Design review of the part built by this model. Coordinates are the model's own, in mm. A direction names the side the tool comes from. Coordinates: 2 decimals unless noted, no trailing zeros. Loops run counter-clockwise (first coordinate to the right, second up) from the corner with the lowest first, then second, coordinate; pieces in that order, holes last. Notation, with made-up numbers: M -3,14 L 38,14 A19 ccw 38,47 Z; hole C -29,-27 d10. An arc over 180 degrees is marked long. Put each result on its own line as item: value. Start each with the question number.
(1) Take a section at B-B, the plane y = -90. Give the boundary of the cut face in (x, z).
(2) Take a section at A-A, the plane x = 180. Give the boundary of the cut face in (y, z).
(3) For probe 1 along X at (y, z) = (-11.5, 4.5); probe 2 along Y at (x, z) = (-180, 4.75); probe 3 along Y at (x, z) = (0, 2.5), list the stretches that pass through material, from the lowest coordinate up. Write a range as [from, to].
(4) For faces 5 (the flat face through (-3, 2, 8)), 6 (the cylindrical face through (110.66, 59.993, 3.944)), list the 3-axis set-ups (+Z, -Z, +X, -X, +Y, -Y) from which the entire face can be reached by the end or side of a thin tool; tool diameter is ignored.
(5) Take a section at C-C, the plane y = -9.5. Give the boundary of the cut face in (x, z).
(6) Take a section at D-D, the plane x = 94. Give the boundary of the cut face in (y, z).
(7) The part is to be moulded in two halves that separate along X. For faces 1 (the flat face through (80, 0, 4)), 2 (the flat face through (-3, 110, 4)), 3 (the cylindrical face through (175.84, -31.72, 3.94)), 4 (the flat face through (-200, -1, 4)), say which applies: +X half, -X half, draft (parallel to the pull), parting line (faces both ways), or undercut.
```python
from build123d import *

# Parameters (mm, degrees)
SKETCH_1_W             = 400
SKETCH_1_H             = 220
EXTRUDE_1_DEPTH        = 8
SKETCH_3_R             = 2.5
SKETCH_3_R_2           = 2.325901808
CUT_EXTRUDE_1_DEPTH    = 10
SKETCH_4_R             = 4.5
CUT_EXTRUDE_2_DEPTH    = 10
CUT_EXTRUDE_3_DEPTH    = 10
HOLE_WIZARD_M8_1_D     = 6.8
HOLE_WIZARD_M8_1_DEPTH = 8
HOLE_WIZARD_M8_2_D     = 6.8
HOLE_WIZARD_M8_2_DEPTH = 8
HOLE_WIZARD_M8_3_D     = 6.8
HOLE_WIZARD_M8_3_DEPTH = 8
CHAMFER_1_SIZE         = 5
SKETCH_12_R            = 4.5
CUT_EXTRUDE_4_DEPTH    = 10


with BuildPart() as part:
    # 草图1 → 凸台-拉伸1 (new body)
    with BuildSketch(Plane.XY):
        Rectangle(SKETCH_1_W, SKETCH_1_H)
    extrude(amount=EXTRUDE_1_DEPTH)

    # 草图3 → 切除-拉伸1 (cut)
    with BuildSketch(Plane.XY.offset(8)):
        with Locations((24, 0)):
            Circle(SKETCH_3_R)
        with Locations((-50, -74)):
            Circle(SKETCH_3_R)
        with Locations((-124, 0)):
            Circle(SKETCH_3_R)
        with Locations((-50, 74)):
            Circle(SKETCH_3_R)
        with Locations((2.325901808, 52.325901808)):
            Circle(SKETCH_3_R_2)
        with Locations((2.325901808, -52.325901808)):
            Circle(SKETCH_3_R_2)
        with Locations((-102.325901808, -52.325901808)):
            Circle(SKETCH_3_R_2)
        with Locations((-102.325901808, 52.325901808)):
            Circle(SKETCH_3_R_2)
    extrude(amount=-CUT_EXTRUDE_1_DEPTH, mode=Mode.SUBTRACT)

    # 草图4 → 切除-拉伸2 (cut)
    with BuildSketch(Plane(origin=(0, 0, 0), x_dir=(-1, 0, 0), z_dir=(0, 0, -1))):
        with Locations((180, 30)):
            Circle(SKETCH_4_R)
        with Locations((180, 90)):
            Circle(SKETCH_4_R)
        with Locations((180, -30)):
            Circle(SKETCH_4_R)
        with Locations((180, -90)):
            Circle(SKETCH_4_R)
        with Locations((-180, -90)):
            Circle(SKETCH_4_R)
        with Locations((-180, -30)):
            Circle(SKETCH_4_R)
        with Locations((-180, 90)):
            Circle(SKETCH_4_R)
        with Locations((-180, 30)):
            Circle(SKETCH_4_R)
    extrude(amount=-CUT_EXTRUDE_2_DEPTH, mode=Mode.SUBTRACT)

    # 草图5 → 切除-拉伸3 (cut)
    with BuildSketch(Plane(origin=(0, 0, 0), x_dir=(-1, 0, 0), z_dir=(0, 0, -1))):
        with BuildLine():
            Line((-80, 30), (-80, -30))
            ThreePointArc((-80, -30), (-110, -60), (-140, -30))
            Line((-140, -30), (-140, 30))
            ThreePointArc((-140, 30), (-110, 60), (-80, 30))
        make_face()
    extrude(amount=-CUT_EXTRUDE_3_DEPTH, mode=Mode.SUBTRACT)

    # M8 螺纹孔1
    with Locations(Plane(origin=(0, 0, 0), x_dir=(-1, 0, 0), z_dir=(0, 0, -1))):
        with Locations((50, 74), (124, 0), (50, -74), (-24, 0)):
            Hole(HOLE_WIZARD_M8_1_D / 2, depth=HOLE_WIZARD_M8_1_DEPTH)

    # M8 螺纹孔2
    with Locations(Plane(origin=(0, 0, 0), x_dir=(-1, 0, 0), z_dir=(0, 0, -1))):
        with Locations((-2.325901808, 52.325901808)):
            Hole(HOLE_WIZARD_M8_2_D / 2, depth=HOLE_WIZARD_M8_2_DEPTH)

    # M8 螺纹孔3
    with Locations(Plane(origin=(0, 0, 0), x_dir=(-1, 0, 0), z_dir=(0, 0, -1))):
        with Locations((102.325901808, 52.325901808), (102.325901808, -52.325901808), (-2.325901808, -52.325901808)):
            Hole(HOLE_WIZARD_M8_3_D / 2, depth=HOLE_WIZARD_M8_3_DEPTH)

    # 倒角1
    chamfer_1_edges = [part.edges().sort_by_distance(p)[0] for p in [
        (-200, 110, 4),
        (200, 110, 4),
        (200, -110, 4),
        (-200, -110, 4),
    ]]
    chamfer(chamfer_1_edges, length=CHAMFER_1_SIZE)

    # 草图12 → 切除-拉伸4 (cut)
    with BuildSketch(Plane(origin=(0, 0, 0), x_dir=(-1, 0, 0), z_dir=(0, 0, -1))):
        with Locations((0, 90)):
            Circle(SKETCH_12_R)
        with Locations((0, -90)):
            Circle(SKETCH_12_R)
    extrude(amount=-CUT_EXTRUDE_4_DEPTH, mode=Mode.SUBTRACT)


solid = part.part
```
Computed values:
1. outline: M -200,0 L -184.5,0 L -184.5,8 L -200,8 Z; M -175.5,0 L -4.5,0 L -4.5,8 L -175.5,8 Z; M 4.5,0 L 175.5,0 L 175.5,8 L 4.5,8 Z; M 184.5,0 L 200,0 L 200,8 L 184.5,8 Z
2. outline: M -110,0 L -94.5,0 L -94.5,8 L -110,8 Z; M -85.5,0 L -34.5,0 L -34.5,8 L -85.5,8 Z; M -25.5,0 L 25.5,0 L 25.5,8 L -25.5,8 Z; M 34.5,0 L 85.5,0 L 85.5,8 L 34.5,8 Z; M 94.5,0 L 110,0 L 110,8 L 94.5,8 Z
3. probe 1: x = [-200, 80], [140, 200]
3. probe 2: y = [-110, -94.5], [-85.5, -34.5], [-25.5, 25.5], [34.5, 85.5], [94.5, 110]
3. probe 3: y = [-110, -94.5], [-85.5, -54.81], [-49.85, 49.85], [54.81, 85.5], [94.5, 110]
4. face 5: +Z, +X, -X, +Y, -Y
4. face 6: +Z, -Z
5. outline: M -200,0 L 80,0 L 80,8 L -200,8 Z; M 140,0 L 200,0 L 200,8 L 140,8 Z
6. outline: M -110,0 L -55.38,0 L -55.38,8 L -110,8 Z; M 55.38,0 L 110,0 L 110,8 L 55.38,8 Z
7. face 1: undercut
7. face 2: draft
7. face 3: undercut
7. face 4: -X half
